Part model, mm, in its own coordinate system. A direction names the side the tool comes from. Give positions to 0.01 mm unless a question says otherwise; leave off trailing zeros. Order: outer loops, then holes, each group sorted by start corner. A loop starts at its lowest first (then second) coordinate and runs counter-clockwise, first axis right, second up. Notation, with made-up numbers: M 4.5,48 L 14.5,48 A20 ccw 14.5,56 Z; hole C 2,49.25 d10. An arc over 180 degrees is marked long. One line per question, with ' | ' between items.
```python
from build123d import *

# Parameters (mm, degrees)
SKETCH_1_W          = 50
SKETCH_1_H          = 20
EXTRUDE_1_DEPTH     = 3
FILLET_1_R          = 10
FILLET_2_R          = 10
FILLET_3_R          = 10
FILLET_4_R          = 10
SKETCH_2_W          = 15
SKETCH_2_H          = 30
EXTRUDE_2_DEPTH     = 3
SKETCH_4_W          = 4
SKETCH_4_H          = 8
EXTRUDE_4_DEPTH     = 7
SKETCH_5_R          = 1.5
CUT_EXTRUDE_1_DEPTH = 58.406445631


with BuildPart() as part:
    # 草图1 → 凸台-拉伸1 (new body)
    with BuildSketch(Plane.XY):
        Rectangle(SKETCH_1_W, SKETCH_1_H)
    extrude(amount=EXTRUDE_1_DEPTH)

    # 圆角1
    fillet_1_edges = [part.edges().sort_by_distance(p)[0] for p in [
        (25, 10, 1.5),
    ]]
    fillet(fillet_1_edges, radius=FILLET_1_R)

    # 圆角2
    fillet_2_edges = [part.edges().sort_by_distance(p)[0] for p in [
        (-25, 10, 1.5),
    ]]
    fillet(fillet_2_edges, radius=FILLET_2_R)

    # 圆角3
    fillet_3_edges = [part.edges().sort_by_distance(p)[0] for p in [
        (25, -10, 1.5),
    ]]
    fillet(fillet_3_edges, radius=FILLET_3_R - 0.0001)  # a hair under: the kernel refuses the full size

    # 圆角4
    fillet_4_edges = [part.edges().sort_by_distance(p)[0] for p in [
        (-25, -10, 1.5),
    ]]
    fillet(fillet_4_edges, radius=FILLET_4_R - 0.0001)  # a hair under: the kernel refuses the full size

    # 草图2 → 凸台-拉伸2 (add)
    with BuildSketch(Plane(origin=(0, 0, 0), x_dir=(-1, 0, 0), z_dir=(0, 0, -1))):
        with Locations((0, -25)):
            Rectangle(SKETCH_2_W, SKETCH_2_H)
    extrude(amount=-EXTRUDE_2_DEPTH)

    # 草图4 → 凸台-拉伸4 (add)
    with BuildSketch(Plane(origin=(0, -40, 0), x_dir=(-1, 0, 0), z_dir=(0, -1, 0))):
        with Locations((-5.5, -1.5)):
            Rectangle(SKETCH_4_W, SKETCH_4_H)
        with Locations((5.5, -1.5)):
            Rectangle(SKETCH_4_W, SKETCH_4_H)
    extrude(amount=EXTRUDE_4_DEPTH)

    # 草图5 → 切除-拉伸1 (cut, through all)
    with BuildSketch(Plane(origin=(7.5, 0, 0), x_dir=(0, 0, -1), z_dir=(1, 0, 0))):
        with Locations(Location((-1.5, -43.5, 0), (0, 0, 180))):
            Circle(SKETCH_5_R)
    extrude(amount=-CUT_EXTRUDE_1_DEPTH, mode=Mode.SUBTRACT)


solid = part.part
```
1. Drop flat-ended pins along their axis: pin 1 (4 mm diameter, centred on x = 15, z = 3.5, fed in from -Y); pin 2 (1 mm diameter, centred on y = -25, z = 4.5, fed in from +X); pin 3 (4 mm diameter, centred on x = 18.5, z = 3, fed in from +Y); pin 4 (3.5 mm diameter, centred on x = 0, z = 1, fed in from -Y). Give the stop position or say it passes through.
Worked out:
pin 1: stops at y = -10 | pin 2: passes through | pin 3: stops at y = 9.89 | pin 4: stops at y = -40
2. Slice it at A-A on z = 3.75. Give the cut face in (x, y), then the cut area to 3 significant figures.
Worked out:
outline: M -7.5,-47 L -3.5,-47 L -3.5,-40 L -7.5,-40 Z; M 3.5,-47 L 7.5,-47 L 7.5,-40 L 3.5,-40 Z | area: 56.0 mm2
3. Probe L1, parallel to Y at x = -5.4, z = 1.5; L2, parallel to Z at x = 5.65, y = -43.5; L3, parallel to X at y = -41, z = 2.25. List the from-to ranges inside material, lowest first. Write a range as from..to.
Worked out:
L1: y = -47..-45, -42..10 | L2: z = -2.5..0, 3..5.5 | L3: x = -7.5..-3.5, 3.5..7.5
4. Slice it at B-B on y = -43.5. Give the cut face in (x, z).
Worked out:
outline: M -7.5,-2.5 L -3.5,-2.5 L -3.5,0 L -7.5,0 Z; M -7.5,3 L -3.5,3 L -3.5,5.5 L -7.5,5.5 Z; M 3.5,-2.5 L 7.5,-2.5 L 7.5,0 L 3.5,0 Z; M 3.5,3 L 7.5,3 L 7.5,5.5 L 3.5,5.5 Z
5. Slice it at D-D on z = 0.75. Give the number of separate pieces and of enclosed holes in the cut face, then the cut area to 3 significant figures.
Worked out:
separate pieces: 3 | enclosed holes: 0 | area: 1,400 mm2
6. Slice it at C-C on x = 4.5. Give the cut face in (y, z), then the cut area to 3 significant figures.
Worked out:
outline: M -47,-2.5 L -40,-2.5 L -40,0 L 10,0 L 10,3 L -40,3 L -40,5.5 L -47,5.5 Z; hole C -43.5,1.5 d3 | area: 199 mm2
7. Mould opens along Z. For faces 4 (the cylindrical face through (5.528, -42.036, 1.175)), 5 (the flat face through (0, -9, 0)), 6 (the flat face through (7.5, -32, 2)) say: released by +Z, released by -Z, zero draft, split by the parting line, or undercut.
Worked out:
face 4: undercut | face 5: released by -Z | face 6: zero draft
8. Tool access for faces 1 (the flat face through (6, -40, 4)), 2 (the flat face through (-3.5, -43.5, -0.2)), 3 (the flat face through (-11, -10, 1)): list every direction of +Z, -Z, +X, -X, +Y, -Y with a clear straight run to the whole face (end or side of a thin tool).
Worked out:
face 1: +Z, +X, -X, +Y | face 2: +Z, -Z, -Y | face 3: +Z, -Z, -X, -Y
